Geometry: final body of the model. Coordinates: model frame, mm. Give positions to 0.01 mm unless a question says otherwise; leave off trailing zeros. Order: outer loops, then holes, each group sorted by start corner. A loop starts at its lowest first (then second) coordinate and runs counter-clockwise, first axis right, second up. Notation, with made-up numbers: (86, 35) - (111, 35) arc R31 ccw to (111, 67) - close; hole circle Ø6 at (-35.5, -19). An arc over 180 degrees is marked (long way). One line per item, written item: value.
Autodesk Inventor part; units mm, degrees
ref_plane "YZ Plane" through (0, 0, 0) normal (1, 0, 0) x (0, 1, 0)
ref_plane "XZ Plane" through (0, 0, 0) normal (0, 1, 0) x (-1, 0, 0)
ref_plane "XY Plane" through (0, 0, 0) normal (0, 0, 1) x (1, 0, 0)
ref_plane "Work Plane1" through (0, 0, 0) normal (0, 0, 1) x (1, 0, 0)
sketch "Sketch1" plane through (0, 0, 0) normal (0, 0, 1) x (1, 0, 0)
  circle A0 centre (-11.2441, 23.3592) radius 16
  circle A1 centre (-11.2441, 23.3592) radius 17
  point P0 (0, 0)
  dimension "d0" = 32
  dimension "d1" = 34
extrude "Extrusion1" add sketch "Sketch1" along normal blind 9
fillet "Fillet1" radius 2 1 edges at (-28.2441, 23.3592, 9)
fillet "Fillet2" radius 2 1 edges at (-28.2441, 23.3592, 0)
properties part number "Tire"
1) Section A-A, the plane z = 8. Return loops of the section in (x, y).
Answers below:
outline: circle Ø33.72 at (-11.24, 23.36); hole circle Ø32 at (-11.24, 23.36)
2) First-contact query: pin 1 (1.5 mm diameter, centred on y = 32.5, z = 4, fed in from +X); pin 2 (10 mm diameter, centred on x = -23, y = 11, fed in from -Z); pin 3 (5 mm diameter, centred on y = 31.5, z = 7, fed in from -X); pin 4 (1 mm diameter, centred on x = 0.5, z = 4, fed in from -Y). Flat tips, straight axial feed; report the tip coordinate or a pass-through.
Answers below:
pin 1: x = 3.54
pin 2: z = 0
pin 3: x = -27.28
pin 4: y = 10.61
3) Material intervals for line 1 along Y through (x, z) = (-2, 2.5); line 2 along X through (y, z) = (24.5, 7); line 3 along X through (y, z) = (37.5, 4.5), sorted ascending.
Answers below:
line 1: 9.09 to 10.3, 36.42 to 37.63
line 2: -28.21 to -27.2, 4.72 to 5.72
line 3: -20.68 to -18.73, -3.76 to -1.81
4) Section B-B, the plane z = 3. Return loops of the section in (x, y), then the cut area to 3 significant figures.
Answers below:
outline: circle Ø34 at (-11.24, 23.36); hole circle Ø32 at (-11.24, 23.36)
area: 104 mm^2
5) Mould query, pull axis Y, two halves, no side actions, for faces 1 (the face through (4.017, 18.553, 4.437)), 2 (the face through (-3.4, 38.44, 4.46)). Classes: released by +Y, released by -Y, zero draft, split by the parting line, or undercut.
Answers below:
face 1: undercut
face 2: split by the parting line
